Check sheet for the modelled part. Datum: model origin and axes. Units: mm. A direction names the side the tool comes from. Coordinates: 2 decimals unless noted, no trailing zeros. Write each loop counter-clockwise with the first axis right and the second up, starting at its lowest first coordinate (ties: lowest second). Pieces come first, ordered by that corner, then holes. Notation, with made-up numbers: (-1.5, 41) -> (11.5, 41) arc R10 cw to (11.5, 46) -> close; hole circle Ø3 at (14, 42.25). An arc over 180 degrees is marked (long way). One line per item, written item: value. Start each with the question number.
1) Sectioned sample at B-B on z = 34. Enter the section's corners in (x, y).
2) Sectioned sample at A-A on x = -17. Enter the section's corners in (y, z), plus the area to 3 significant figures.
3) Draft check along Z on faces 6 (the cylindrical face through (-61.94, -0.99, -51.98)), 7 (the cylindrical face through (-60.19, 0.76, 48.58)), 8 (the flat face through (68, 1, -1)), 9 (the cylindrical face through (66.196, 1.479, -56.289)). Enter one of: +Z half, -Z half, draft (parallel to the pull), parting line (faces both ways), or undercut.
4) Set-up check for faces 1 (the cylindrical face through (-63.98, -0.99, -53.94)), 2 (the cylindrical face through (61.94, -0.99, 51.98)), 3 (the flat face through (-68, 1, 1)), 4 (the cylindrical face through (63.98, -0.99, 53.94)), 5 (the cylindrical face through (63.94, -0.99, -53.98)): record each of +Z, -Z, +X, -X, +Y, -Y from which the full face is reachable in a straight line by a thin tool's end or side.
5) Scan lines: line 1 along Z through (x, y) = (60.09, 0.55); line 2 along X through (y, z) = (0.95, -50.2); line 3 along Z through (x, y) = (59.5, -1.3). Record each from-to range of solid material in increasing order. Write a range as [from, to].
6) Gauge pin test, flat ends, axial feed: P1, Ø3, axis at x = -39.5, z = -24.5, coming from the -Y side; P2, Ø5.5, axis at x = -60.7, z = -50.2, coming from the +Y side; P3, Ø0.6, axis at y = -1, z = 22.5, coming from the -X side; P4, Ø2.5, axis at x = -60.7, z = 50.2, coming from the -Y side. Record the tip position at first contact, or that the pin passes through.
```python
from build123d import *

# Parameters (mm, degrees)
BOSS_EXTRUDE1_DEPTH                                 = 3
BOSS_EXTRUDE2_DEPTH                                 = 5
CSK_FOR_M3_COUNTERSUNK_FLAT_HEAD_SCREW1_D           = 3.4
CSK_FOR_M3_COUNTERSUNK_FLAT_HEAD_SCREW1_DEPTH       = 6
CSK_FOR_M3_COUNTERSUNK_FLAT_HEAD_SCREW1_CSINK_D     = 6.3
CSK_FOR_M3_COUNTERSUNK_FLAT_HEAD_SCREW1_CSINK_ANGLE = 90
CSK_FOR_M3_COUNTERSUNK_FLAT_HEAD_SCREW1_TIP         = 1.021463052


with BuildPart() as part:
    # Sketch1 → Boss-Extrude1 (new body)
    with BuildSketch(Plane(origin=(0, 0, 0), x_dir=(1, 0, 0), z_dir=(0, 1, 0))):
        with BuildLine():
            Line((62, -58), (-62, -58))
            ThreePointArc((-62, -58), (-66.242640687, -56.242640687), (-68, -52))
            Line((-68, -52), (-68, 52))
            ThreePointArc((-68, 52), (-66.242640687, 56.242640687), (-62, 58))
            Line((-62, 58), (62, 58))
            ThreePointArc((62, 58), (66.242640687, 56.242640687), (68, 52))
            Line((68, 52), (68, -52))
            ThreePointArc((68, -52), (66.242640687, -56.242640687), (62, -58))
        make_face()
    extrude(amount=BOSS_EXTRUDE1_DEPTH)

    # Sketch2 → Boss-Extrude2 (add)
    with BuildSketch(Plane(origin=(0, 3, 0), x_dir=(1, 0, 0), z_dir=(0, 1, 0))):
        with BuildLine():
            Line((-61.84, 54.84), (61.84, 54.84))
            ThreePointArc((61.84, 54.84), (63.961320344, 53.961320344), (64.84, 51.84))
            Line((64.84, 51.84), (64.84, -51.84))
            ThreePointArc((64.84, -51.84), (63.961320344, -53.961320344), (61.84, -54.84))
            Line((61.84, -54.84), (-61.84, -54.84))
            ThreePointArc((-61.84, -54.84), (-63.961320344, -53.961320344), (-64.84, -51.84))
            Line((-64.84, -51.84), (-64.84, 51.84))
            ThreePointArc((-64.84, 51.84), (-63.961320344, 53.961320344), (-61.84, 54.84))
        make_face()
        with BuildLine():
            Line((-62.84, 49.84), (-62.84, -49.84))
            ThreePointArc((-62.84, -49.84), (-61.961320344, -51.961320344), (-59.84, -52.84))
            Line((-59.84, -52.84), (59.84, -52.84))
            ThreePointArc((59.84, -52.84), (61.961320344, -51.961320344), (62.84, -49.84))
            Line((62.84, -49.84), (62.84, 49.84))
            ThreePointArc((62.84, 49.84), (61.961320344, 51.961320344), (59.84, 52.84))
            Line((59.84, 52.84), (-59.84, 52.84))
            ThreePointArc((-59.84, 52.84), (-61.961320344, 51.961320344), (-62.84, 49.84))
        make_face(mode=Mode.SUBTRACT)
    extrude(amount=-BOSS_EXTRUDE2_DEPTH)

    # CSK for M3 Countersunk Flat Head Screw1
    with Locations(Plane(origin=(-60.7, 3, -50.2), x_dir=(0, 0, 1), z_dir=(0, 1, 0))):
        with Locations((0, 0), (0, 60.74), (0, 120.79), (100.4, 0), (100.4, 60.74), (100.4, 120.79)):
            CounterSinkHole(CSK_FOR_M3_COUNTERSUNK_FLAT_HEAD_SCREW1_D / 2, CSK_FOR_M3_COUNTERSUNK_FLAT_HEAD_SCREW1_CSINK_D / 2, depth=CSK_FOR_M3_COUNTERSUNK_FLAT_HEAD_SCREW1_DEPTH, counter_sink_angle=CSK_FOR_M3_COUNTERSUNK_FLAT_HEAD_SCREW1_CSINK_ANGLE)
            with Locations((0, 0, -(CSK_FOR_M3_COUNTERSUNK_FLAT_HEAD_SCREW1_DEPTH + CSK_FOR_M3_COUNTERSUNK_FLAT_HEAD_SCREW1_TIP / 2))):  # 118° drill point
                Cone(0, CSK_FOR_M3_COUNTERSUNK_FLAT_HEAD_SCREW1_D / 2, CSK_FOR_M3_COUNTERSUNK_FLAT_HEAD_SCREW1_TIP, mode=Mode.SUBTRACT)


solid = part.part
```
Answers:
1. outline: (-68, 0) -> (-64.84, 0) -> (-64.84, -2) -> (-62.84, -2) -> (-62.84, 0) -> (62.84, 0) -> (62.84, -2) -> (64.84, -2) -> (64.84, 0) -> (68, 0) -> (68, 3) -> (-68, 3) -> close
2. outline: (-2, -54.84) -> (0, -54.84) -> (0, -58) -> (3, -58) -> (3, 58) -> (0, 58) -> (0, 54.84) -> (-2, 54.84) -> (-2, 52.84) -> (0, 52.84) -> (0, -52.84) -> (-2, -52.84) -> close
2. area: 356 mm2
3. face 6: undercut
3. face 7: undercut
3. face 8: draft
3. face 9: -Z half
4. face 1: -Z, -X, -Y
4. face 2: -Y
4. face 3: +Z, -Z, -X, +Y, -Y
4. face 4: +Z, +X, -Y
4. face 5: -Z, +X, -Y
5. line 1: z = [-58, -51.9], [-48.5, 48.5], [51.9, 58]
5. line 2: x = [-68, -62.4], [-59, -1.66], [1.74, 58.39], [61.79, 68]
5. line 3: z = [-54.84, -52.84], [52.84, 54.84]
6. P1: stops at y = 0
6. P2: stops at y = 2.6
6. P3: stops at x = -64.84
6. P4: passes through
